Geometry: final body of the model. Coordinates: model frame, mm. Face numbers are marked on the shaded views. A direction names the side the tool comes from. Give positions to 0.01 mm unless a question says otherwise; leave off trailing zeros. Loops run counter-clockwise (first coordinate to the right, second up) from the corner with the lowest first, then second, coordinate; pieces in that order, holes last. Notation, with made-up numbers: (26.5, 19.25) - (62.5, 19.25) arc R24 ccw to (62.5, 39.25) - close; hole circle Ø9 at (-20, -30). An arc over 180 degrees is marked (long way). Use one line per item in the form item = value.
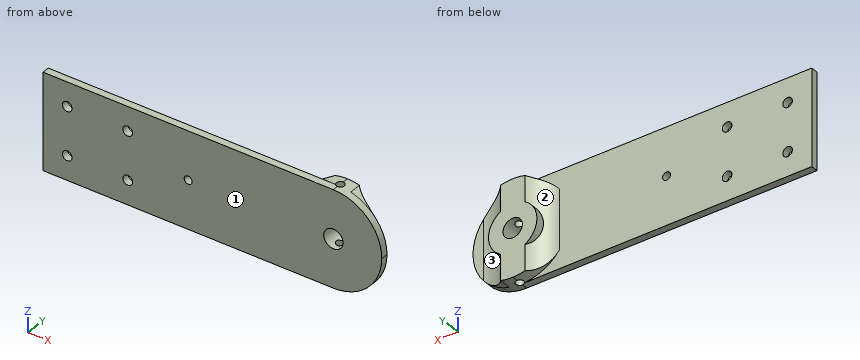
```python
from build123d import *

# Parameters (mm, degrees)
SKETCH1_R           = 2
SKETCH1_R_2         = 4
BOSS_EXTRUDE1_DEPTH = 8
CUT_EXTRUDE1_START  = -5
SKETCH4_R           = 2
CUT_EXTRUDE1_DEPTH  = 5
FILLET2_R           = 14
M4_TAPPED_HOLE1_D   = 3.3
SKETCH5_R           = 1.65
CUT_EXTRUDE2_DEPTH  = 122.757956639
CUT_EXTRUDE3_START  = -5
CUT_EXTRUDE3_DEPTH  = 5


with BuildPart() as part:
    # Sketch1 → Boss-Extrude1 (new body)
    with BuildSketch(Plane(origin=(0, 0, 0), x_dir=(1, 0, 0), z_dir=(0, 1, 0))):
        with BuildLine():
            Line((0, 20), (-120, 20))
            Line((-120, 20), (-120, -5))
            Line((-120, -5), (-120, -20))
            Line((-120, -20), (0, -20))
            ThreePointArc((0, -20), (14.142135607, -14.14213564), (20, -4.7e-08))
            ThreePointArc((20, -4.7e-08), (14.14213564, 14.142135607), (0, 20))
        make_face()
        with Locations(Location((-110, -10, 0), (0, 0, 270))):
            Circle(SKETCH1_R, mode=Mode.SUBTRACT)
        with Locations(Location((-85, -10, 0), (0, 0, 270))):
            Circle(SKETCH1_R, mode=Mode.SUBTRACT)
        with Locations(Location((-110, 10, 0), (0, 0, 270))):
            Circle(SKETCH1_R, mode=Mode.SUBTRACT)
        with Locations(Location((-85, 10, 0), (0, 0, 270))):
            Circle(SKETCH1_R, mode=Mode.SUBTRACT)
        with Locations(Location((0, 0, 0), (0, 0, 270))):
            Circle(SKETCH1_R_2, mode=Mode.SUBTRACT)
    extrude(amount=BOSS_EXTRUDE1_DEPTH)

    # Sketch4 → Cut-Extrude1 (cut)
    # profile 1 of 2: a face of its own
    with BuildSketch(Plane(origin=(0, 8, 0), x_dir=(1, 0, 0), z_dir=(0, 1, 0)).offset(CUT_EXTRUDE1_START)):
        with BuildLine():
            Line((-5, 8.660254038), (-5, 20))
            Line((-5, 20), (-120, 20))
            Line((-120, 20), (-120, -20))
            Line((-120, -20), (-5, -20))
            Line((-5, -20), (-5, -8.660254038))
            ThreePointArc((-5, -8.660254038), (-10, 0), (-5, 8.660254038))
        make_face()
        with Locations(Location((-110, -10, 0), (0, 0, 270))):
            Circle(SKETCH4_R, mode=Mode.SUBTRACT)
        with Locations(Location((-85, -10, 0), (0, 0, 270))):
            Circle(SKETCH4_R, mode=Mode.SUBTRACT)
        with Locations(Location((-110, 10, 0), (0, 0, 270))):
            Circle(SKETCH4_R, mode=Mode.SUBTRACT)
        with Locations(Location((-85, 10, 0), (0, 0, 270))):
            Circle(SKETCH4_R, mode=Mode.SUBTRACT)
    # profile 2 of 2: a face of its own
    with BuildSketch(Plane(origin=(0, 8, 0), x_dir=(1, 0, 0), z_dir=(0, 1, 0)).offset(CUT_EXTRUDE1_START)):
        with BuildLine():
            ThreePointArc((5, -19.364916731), (20, 0), (5, 19.364916731))
            Line((5, 19.364916731), (5, 8.660254038))
            ThreePointArc((5, 8.660254038), (10, 0), (5, -8.660254038))
            Line((5, -8.660254038), (5, -19.364916731))
        make_face()
    extrude(amount=CUT_EXTRUDE1_DEPTH, mode=Mode.SUBTRACT)

    # Fillet2
    # the kernel refuses this fillet: 14 mm, written as the material it adds along each edge
    with BuildSketch(Plane(origin=(-5, 3, 20), x_dir=(-1, 0, 0), z_dir=(0, 0, -1)), Plane(origin=(-5, 3, 18.149259199), x_dir=(-1, 0, 0), z_dir=(0, 0, -1))) as fillet2_piece_1:
        with BuildLine():
            CenterArc((10.723805295, 14), FILLET2_R, 220.005200885, 49.994799115)
            Line((0, 5), (0, 0))
            Line((0, 0), (10.723805295, 0))
        make_face()
    extrude(amount=38.149259199)
    with BuildSketch(Plane(origin=(5, 3, -46.174429968), x_dir=(0, 1, 0), z_dir=(0, 0, 1))) as fillet2_piece_2_section:
        with BuildLine():
            CenterArc((14, -10.723805295), FILLET2_R, 130.005200885, 49.994799115)
            Line((0, -10.723805295), (0, 0))
            Line((0, 0), (5, 0))
        make_face()
    fillet2_piece_2 = extrude(amount=64.323689167, mode=Mode.PRIVATE)
    fillet2_piece_2 = fillet2_piece_2 & Plane(origin=(0, 3, 0), x_dir=(0, 0, 1), z_dir=(0, -1, 0)) * Cylinder(20, 172, mode=Mode.PRIVATE)
    add(fillet2_piece_2)
    with BuildSketch(Plane(origin=(5, 3, -18.149259199), x_dir=(0, 1, 0), z_dir=(0, 0, 1))) as fillet2_piece_3_section:
        with BuildLine():
            CenterArc((14, -10.723805295), FILLET2_R, 130.005200885, 49.994799115)
            Line((0, -10.723805295), (0, 0))
            Line((0, 0), (5, 0))
        make_face()
    fillet2_piece_3 = extrude(amount=64.323689167, mode=Mode.PRIVATE)
    fillet2_piece_3 = fillet2_piece_3 & Plane(origin=(0, 3, 0), x_dir=(0, 0, 1), z_dir=(0, -1, 0)) * Cylinder(20, 172, mode=Mode.PRIVATE)
    add(fillet2_piece_3)

    # M4 Tapped Hole1 (through all)
    with Locations(Plane(origin=(0, 0, -20), x_dir=(-1, 0, 0), z_dir=(0, 0, -1))):
        with Locations((0, 4)):
            Hole(M4_TAPPED_HOLE1_D / 2)

    # Sketch5 → Cut-Extrude2 (cut, through all)
    with BuildSketch(Plane(origin=(0, 3, 0), x_dir=(1, 0, 0), z_dir=(0, 1, 0))):
        with Locations(Location((-60, 0, 0), (0, 0, 270))):
            Circle(SKETCH5_R)
    extrude(amount=-CUT_EXTRUDE2_DEPTH, mode=Mode.SUBTRACT)

    # Sketch6 → Cut-Extrude3 (cut)
    with BuildSketch(Plane(origin=(0, 8, 0), x_dir=(1, 0, 0), z_dir=(0, 1, 0)).offset(CUT_EXTRUDE3_START)):
        with BuildLine():
            Line((-120, -20), (0, -20))
            ThreePointArc((0, -20), (-20, 0), (0, 20))
            Line((0, 20), (-120, 20))
            Line((-120, 20), (-120, -20))
        make_face()
    extrude(amount=CUT_EXTRUDE3_DEPTH, mode=Mode.SUBTRACT)


solid = part.part
```
(1) Material intervals for L1, parallel to X at y = 2.15, z = -10; L2, parallel to Y at x = 0, z = 11; L3, parallel to Y at x = -69.5, z = 12.5, sorted ascending. Write a range as from..to.
Solution:
L1 = -120..-112, -108..-87, -83..17.32
L2 = 0..2.35, 5.65..8
L3 = 0..3
(2) Access query for the marked faces 1, 2 and 3. Directions: +Z, -Z, +X, -X, +Y, -Y. A direction counts if a zero-diameter tool reaches every point of the face in a straight line with its end or side. Return the directions, or none.
Solution:
face_1 = +Z, -Z, +X, -X, -Y
face_2 = -X, +Y
face_3 = +X, +Y
(3) Cut plane A-A (x = -110). Return the cut outline in (y, z), plus the area to 3 significant figures.
Solution:
outline = (0, -20) - (3, -20) - (3, -12) - (0, -12) - close; (0, -8) - (3, -8) - (3, 8) - (0, 8) - close; (0, 12) - (3, 12) - (3, 20) - (0, 20) - close
area = 96.0 mm2
(4) Cut plane B-B (z = -10). Return the cut outline in (x, y), plus the area to 3 significant figures.
Solution:
outline = (-120, 0) - (-112, 0) - (-112, 3) - (-120, 3) - close; (-108, 0) - (-87, 0) - (-87, 3) - (-108, 3) - close; (-83, 0) - (17.32, 0) - (17.32, 3) - (15.72, 3) arc R14 cw to (5, 8) - (-5, 8) arc R14 cw to (-15.72, 3) - (-83, 3) - close; hole circle Ø3.3 at (0, 4)
area = 462 mm2
(5) Pin query (flat end, axial travel): P1, Ø4.5, axis at x = -85, z = 10, coming from the +Y side; P2, Ø3.5, axis at x = -85, z = -10, coming from the +Y side. Return the tip coordinate at first contact, or that it passes through.
Solution:
P1 = 3
P2 = through
